Here's the drawing with two shaded views (mm, measured from the low corner). I have some questions. A direction names the side the tool comes from. Round coordinates to 2 decimals unless told otherwise and drop trailing zeros. Loops run counter-clockwise (first coordinate to the right, second up) from the corner with the lowest first, then second, coordinate; pieces in that order, holes last. Notation, with made-up numbers: (10.25, -33.5) - (60.25, -33.5) arc R15 ccw to (60.25, -11.5) - close; hole circle Ø2 at (48.5, -13.5). An arc over 180 degrees is marked (long way). Use one line per item in the form item = value.
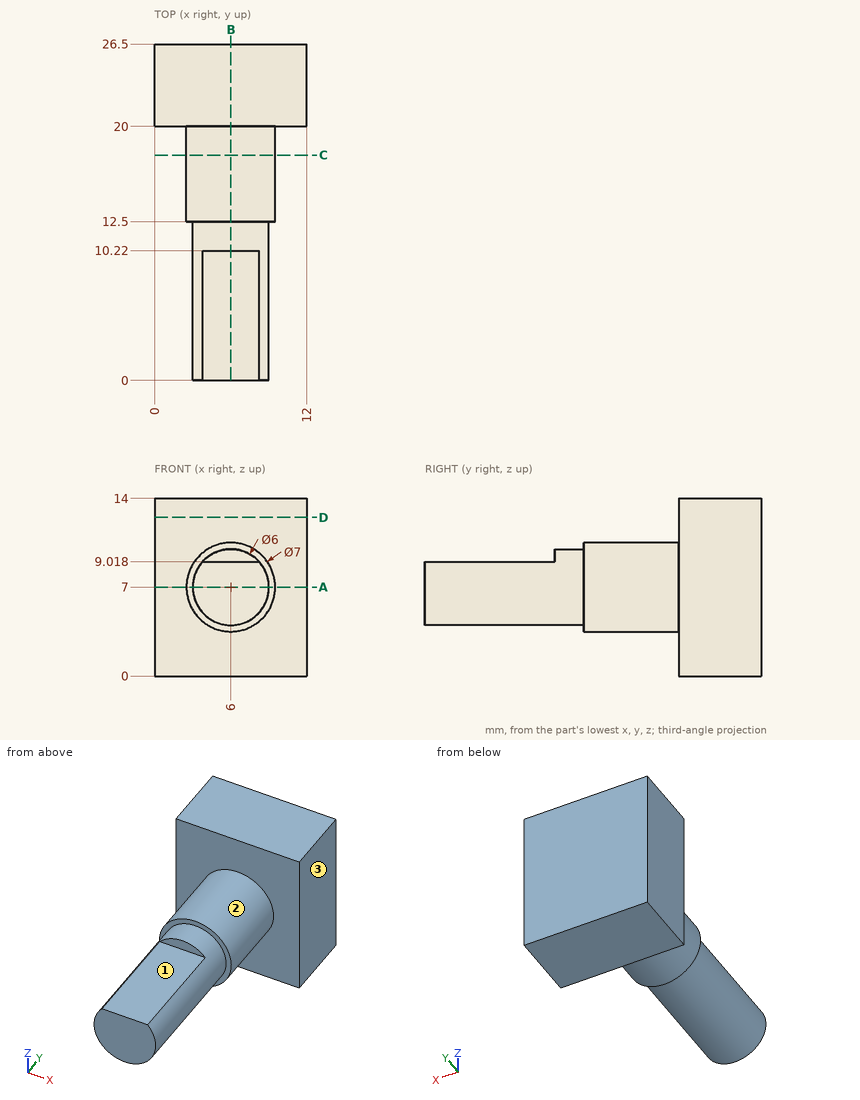
1. For P1, Ø4, axis at y = 4, z = 4.5, coming from the +X side; P2, Ø2, axis at x = 6, y = 5.5, coming from the +Z side; P3, Ø1, axis at x = 3.5, y = 15, coming from the -Z side, each with a flat end and sliding along its axis, tell me the tip position at first contact or that it passes through.
Solution:
P1 = 8.96
P2 = 9.02
P3 = 4.13
2. On a 3-axis mill with a long thin cutter (end or side, diameter ignored), from which of +Z, -Z, +X, -X, +Y, -Y can I reach the whole of each face in a straight line? I mean the marked faces 1, 2 and 3. Say none if no direction works.
Solution:
face_1 = +Z, +X, -X, -Y
face_2 = -Y
face_3 = +Z, -Z, +X, +Y, -Y
3. If we section it at A-A, the plane z = 7: Write out the boundary of the cut face in (x, y).
Solution:
outline = (0, 20) - (2.5, 20) - (2.5, 12.5) - (3, 12.5) - (3, 0) - (9, 0) - (9, 12.5) - (9.5, 12.5) - (9.5, 20) - (12, 20) - (12, 26.5) - (0, 26.5) - close
4. If we section it at C-C, the plane y = 17.75: Write out the boundary of the cut face in (x, z), plus the area to 3 significant figures.
Solution:
outline = circle Ø7 at (6, 7)
area = 38.5 mm^2
5. If we section it at D-D, the plane z = 12.5: Write out the boundary of the cut face in (x, y), plus the area to 3 significant figures.
Solution:
outline = (0, 20) - (12, 20) - (12, 26.5) - (0, 26.5) - close
area = 78.0 mm^2
6. Please list where these lines run through material, in increasing order: line 1 along Y through (x, z) = (7.5, 1.75); line 2 along X through (y, z) = (12.75, 7.5) (1 decimal); line 3 along X through (y, z) = (8.25, 8.75) (1 decimal).
Solution:
line_1 = 20 to 26.5
line_2 = 2.5 to 9.5
line_3 = 3.6 to 8.4
7. If we section it at B-B, the plane x = 6: Write out the boundary of the cut face in (y, z).
Solution:
outline = (0, 4) - (12.5, 4) - (12.5, 3.5) - (20, 3.5) - (20, 0) - (26.5, 0) - (26.5, 14) - (20, 14) - (20, 10.5) - (12.5, 10.5) - (12.5, 10) - (10.22, 10) - (10.22, 9.02) - (0, 9.02) - close
